Geometry check sheet. Reference: the model listing, model coordinates, mm. Round coordinates to 2 decimals unless told otherwise and drop trailing zeros. Write each loop counter-clockwise with the first axis right and the second up, starting at its lowest first coordinate (ties: lowest second). Pieces come first, ordered by that corner, then holes. Notation, with made-up numbers: M 9,71.5 L 39,71.5 A29 cw 39,104.5 Z; hole C 76.25,-14.75 d2. An arc over 180 degrees is marked long. Answer as CSV lines item,"result". Start each with the question number.
Autodesk Inventor part; units mm, degrees
ref_plane "YZ Plane" through (0, 0, 0) normal (1, 0, 0) x (0, 1, 0)
ref_plane "XZ Plane" through (0, 0, 0) normal (0, 1, 0) x (-1, 0, 0)
ref_plane "XY Plane" through (0, 0, 0) normal (0, 0, 1) x (1, 0, 0)
sketch "Sketch1" plane through (0, 0, 0) normal (0, 0, 1) x (1, 0, 0)
  circle A0 centre (0, 0) radius 38.1 construction
  circle A1 centre (-41.3753, -19.4526) radius 7.62 construction
  circle A2 centre (-19.4526, 41.3753) radius 7.62 construction
  circle A3 centre (41.3753, 19.4526) radius 7.62 construction
  circle A4 centre (-41.3753, -19.4526) radius 29.972 construction
  circle A5 centre (-19.4526, 41.3753) radius 29.972 construction
  circle A6 centre (41.3753, 19.4526) radius 29.972 construction
  line L0 (-31.2131, 8.7441) -> (-29.6148, 13.1787) construction
  line L1 (8.7441, 31.2131) -> (13.1787, 29.6148) construction
  circle A7 centre (0, 0) radius 19.05 construction
  circle A8 centre (53.1378, -12.5946) radius 35.56 construction
  circle A9 centre (53.1378, -12.5946) radius 14.2875
  circle A10 centre (41.3753, 19.4526) radius 10.3251
  line L2 (44.9329, 9.7597) -> (48.2149, 0.818) construction
  circle A11 centre (53.1378, -12.5946) radius 36.83 construction
  line L3 (-41.3753, -49.4246) -> (53.1378, -49.4246)
  circle A12 centre (-19.4526, 41.3753) radius 10.3251
  circle A13 centre (-41.3753, -19.4526) radius 10.3251
  circle A14 centre (21.029, -43.7899) radius 6.35 construction
  circle A15 centre (0, 0) radius 40.64 construction
  line L4 (-7.2269, -37.4083) -> (-7.7087, -39.9022) construction
  circle A16 centre (21.029, -43.7899) radius 2.4892
  line L5 (18.2801, -38.0657) -> (17.5929, -36.6347) construction
  line L6 (25.5834, -39.365) -> (26.722, -38.2588) construction
  circle A17 centre (-49.0395, 17.6741) radius 6.35 construction
  circle A18 centre (-49.0395, 17.6741) radius 2.4892
  circle A19 centre (17.6741, 49.0395) radius 6.35 construction
  circle A20 centre (17.6741, 49.0395) radius 2.4892
  circle A21 centre (79.0191, 23.9334) radius 2.4892
  circle A22 centre (79.0191, 23.9334) radius 6.35 construction
  line L7 (-47.7557, 11.4552) -> (-47.4347, 9.9005) construction
  line L8 (-44.0835, 21.6442) -> (-42.8445, 22.6367) construction
  line L9 (11.4552, 47.7557) -> (9.9005, 47.4347) construction
  line L10 (21.6442, 44.0835) -> (22.6367, 42.8445) construction
  line L11 (72.7136, 23.1828) -> (71.1372, 22.9952) construction
  line L12 (75.348, 18.7521) -> (74.4302, 17.4568) construction
  line L13 (-69.5719, -9.2903) -> (-47.6492, 51.5375)
  arc A23 (-69.5719, -9.2903) -> (-41.3753, -49.4246) centre (-41.3753, -19.4526) ccw
  line L14 (-9.2903, 69.5719) -> (51.5375, 47.6492)
  arc A24 (-9.2903, 69.5719) -> (-47.6492, 51.5375) centre (-19.4526, 41.3753) ccw
  line L15 (57.1496, 44.9377) -> (82.3611, 29.3328)
  line L16 (85.3134, 24.7723) -> (89.645, -7.7291)
  arc A25 (57.1496, 44.9377) -> (51.5375, 47.6492) centre (41.3753, 19.4526) ccw
  arc A26 (85.3134, 24.7723) -> (82.3611, 29.3328) centre (79.0191, 23.9334) ccw
  arc A27 (53.1378, -49.4246) -> (89.645, -7.7291) centre (53.1378, -12.5946) ccw
  circle A28 centre (0, 0) radius 14.2875
  dimension "d0" = 76.2
  dimension "d5" = 28.575
  dimension "d6" = 20.6502
  dimension "d1" = 15.24
  dimension "d2" = 59.944
  dimension "d3" = 38.1
  dimension "d4" = 71.12
  dimension "d8" = 9.525
  dimension "d9" = 73.66
  dimension "d10" = 2.54
  dimension "d12" = 12.7
  dimension "d13" = 4.9784
  dimension "d14" = 1.5875
  dimension "d15" = 12.7
  dimension "d16" = 4.9784
  dimension "d17" = 12.7
  dimension "d18" = 4.9784
  dimension "d19" = 12.7
  dimension "d20" = 4.9784
  dimension "d21" = 1.5875
  dimension "d22" = 1.5875
  dimension "d23" = 1.5875
  dimension "d24" = 1.5875
extrude "Extrusion1" add sketch "Sketch1" along normal blind 4.7625
properties part number "bottomplate_gearbox4" material "Aluminum 6061"
1) Section check A-A, the plane x = 0. Record the cut outline in (y, z).
2) Scan lines: line 1 (X direction, y = -17, z = 0.9); line 2 (X direction, y = 10, z = 3.9); line 3 (Y direction, x = -6.5, z = 0.85). Record each from-to range of solid material in increasing order. Write a range as from..to.
3) Section check C-C, the plane x = 48.5. Record the cut outline in (y, z), plus the area to 3 significant figures.
4) Go/stop test with flat-tipped pins: pin 1 (12 mm diameter, centred on x = -13.5, y = -10.5, fed in from -Z); pin 2 (4.5 mm diameter, centred on x = -49.04, y = 17.67, fed in from -Z); pin 3 (1.5 mm diameter, centred on y = 26.5, z = 2.5, fed in from +X). Record where each tip stops, or that it passes through.
5) Section check D-D, the plane z = 2.05. Give the number of separate pieces and of enclosed holes in the cut face, plus the area to 3 significant figures.
6) Section check B-B, the plane y = 0. Record the cut outline in (x, z), plus the area to 3 significant figures.
7) Mould release check, pull along X, two halves, no side actions. Record for faces 1 (the flat face through (-58.764, 20.698, 2.348)), 2 (the cylindrical face through (-47.701, 15.575, 2.348)), 3 (the cylindrical face through (81.135, -36.524, 2.348)): released by +X, released by -X, zero draft, split by the parting line, or undercut.
Results:
1,outline,"M -49.42,0 L -14.29,0 L -14.29,4.76 L -49.42,4.76 Z; M 14.29,0 L 66.22,0 L 66.22,4.76 L 14.29,4.76 Z"
2,line 1,"x = -71.25..-51.4, -31.35..39.55, 66.73..89.7"
2,line 2,"x = -62.62..-10.2, 10.2..37.22, 45.53..87.28"
2,line 3,"y = -49.42..-12.72, 12.72..68.57"
3,outline,"M -49.42,0 L -26.11,0 L -26.11,4.76 L -49.42,4.76 Z; M 0.92,0 L 11.98,0 L 11.98,4.76 L 0.92,4.76 Z; M 26.93,0 L 48.74,0 L 48.74,4.76 L 26.93,4.76 Z"
3,area,"268 mm^2"
4,pin 1,"stops at z = 0"
4,pin 2,"passes through"
4,pin 3,"stops at x = 85.1"
5,separate pieces,"1"
5,enclosed holes,"9"
5,area,"13,000 mm^2"
6,outline,"M -66.22,0 L -14.29,0 L -14.29,4.76 L -66.22,4.76 Z; M 14.29,0 L 46.39,0 L 46.39,4.76 L 14.29,4.76 Z; M 59.88,0 L 88.61,0 L 88.61,4.76 L 59.88,4.76 Z"
6,area,"537 mm^2"
7,face 1,"released by -X"
7,face 2,"undercut"
7,face 3,"released by +X"
